Geometry: see drawing. Coordinates: mm, zero at the bounding-box minimum. A direction names the side the tool comes from. Give positions to 0.01 mm unless a question says otherwise; leave off trailing zeros. Write each loop counter-clockwise with the first axis right and the second up, starting at its lowest first coordinate (ties: lowest second). Pieces come first, ordered by that corner, then holes. Notation, with made-up numbers: (-39, 76) -> (-5, 76) arc R36 ccw to (-5, 112) -> close; hole circle Ø2 at (35.5, 31.25). An arc over 180 degrees is marked (long way). Answer as a JSON object with one key per item and string values. Group by question number.
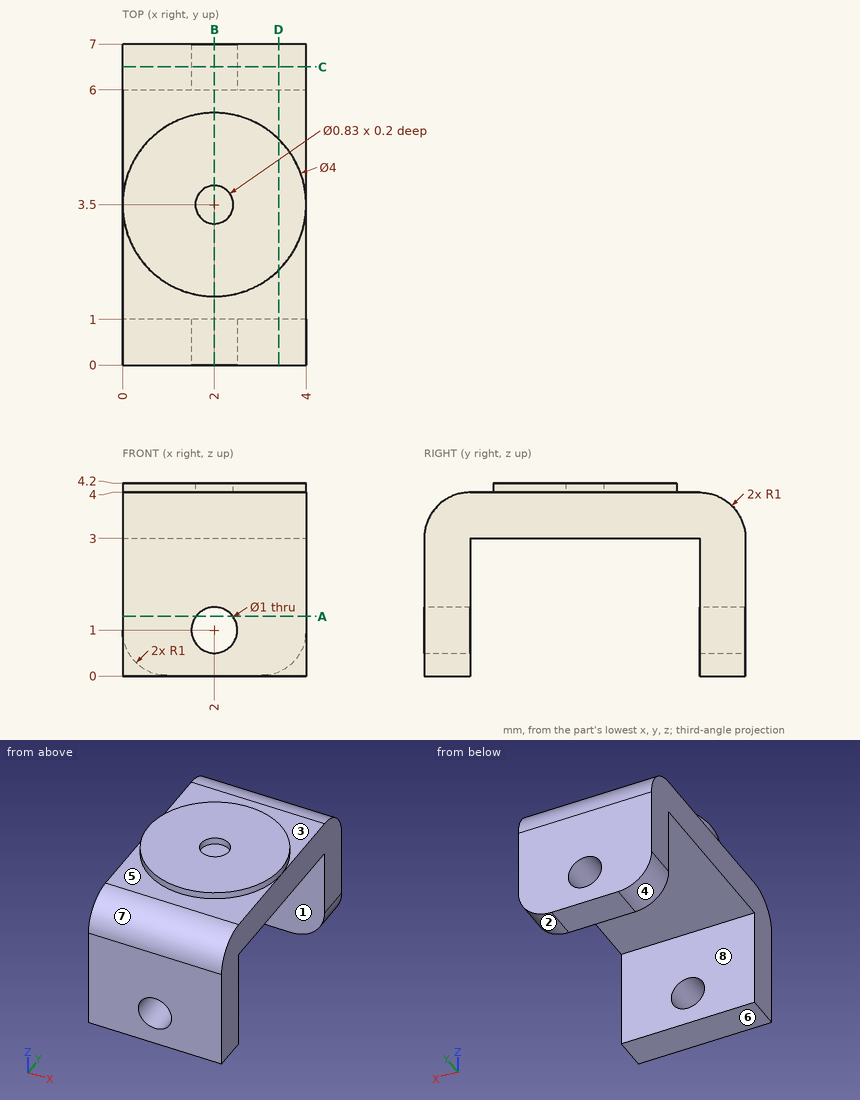
1. Line query: line 1 (Y direction, x = 0.65, z = 2.4); line 2 (Y direction, x = 2, z = 4.15) (3 decimals); line 3 (X direction, y = 0.65, z = 1). Output: solid intervals per line, ascending.
2. Contact query for flat-ended pins moving along their axis: pin 1 Ø1.2 at (x, y) = (1, 4) entering from -Z; pin 2 Ø2 at (y, z) = (4, 1.5) entering from +X. Output: stop coordinate, or through.
3. Mould query, pull axis Y, two halves, no side actions, for the marked faces 6, 7 and 8. Classes: pulls with the +Y half, pulls with the -Y half, needs draft (parallel to the pull), parting line crosses it, or undercut.
4. Reachability of the marked faces 1, 2, 3, 4 and 5 from +Z, -Z, +X, -X, +Y, -Y: full face, straight path, thin tool, end or side. Return the list, or none.
5. Section A-A (z = 1.3). Return the cut outline in (x, y).
6. Section D-D (x = 3.4). Return the cut outline in (y, z), plus the area to 3 significant figures.
7. Section C-C (y = 6.5). Return the cut outline in (x, z), plus the area to 3 significant figures.
8. Section B-B (x = 2). Return the cut outline in (y, z) (3 decimals), plus the area to 3 significant figures.
Working result:
{
 "1": {"line 1": "y = 0 to 1, 6 to 7", "line 2": "y = 1.5 to 3.085, 3.915 to 5.5", "line 3": "x = 0 to 1.5, 2.5 to 4"},
 "2": {"pin 1": "stops at z = 3", "pin 2": "passes through"},
 "3": {"face 6": "needs draft", "face 7": "pulls with the -Y half", "face 8": "undercut"},
 "4": {"face 1": "-Z, +X, -X", "face 2": "-Z, +X, +Y", "face 3": "+Z, +Y", "face 4": "-Z, -X, +Y", "face 5": "+Z, -Y"},
 "5": {"outline": "(0, 0) -> (1.6, 0) -> (1.6, 1) -> (0, 1) -> close; (0, 6) -> (1.6, 6) -> (1.6, 7) -> (0, 7) -> close; (2.4, 0) -> (4, 0) -> (4, 1) -> (2.4, 1) -> close; (2.4, 6) -> (4, 6) -> (4, 7) -> (2.4, 7) -> close"},
 "6": {"outline": "(0, 0) -> (1, 0) -> (1, 3) -> (6, 3) -> (6, 0.08) -> (7, 0.08) -> (7, 3) arc R1 ccw to (6, 4) -> (4.93, 4) -> (4.93, 4.2) -> (2.07, 4.2) -> (2.07, 4) -> (1, 4) arc R1 ccw to (0, 3) -> close", "area": "13.1 mm^2"},
 "7": {"outline": "(0, 1) arc R1 ccw to (1, 0) -> (3, 0) arc R1 ccw to (4, 1) -> (4, 3.87) -> (0, 3.87) -> close; hole circle Ø1 at (2, 1)", "area": "14.2 mm^2"},
 "8": {"outline": "(0, 0) -> (1, 0) -> (1, 0.5) -> (0, 0.5) -> close; (0, 1.5) -> (1, 1.5) -> (1, 3) -> (6, 3) -> (6, 1.5) -> (7, 1.5) -> (7, 3) arc R1 ccw to (6, 4) -> (5.5, 4) -> (5.5, 4.2) -> (3.915, 4.2) -> (3.915, 4) -> (3.085, 4) -> (3.085, 4.2) -> (1.5, 4.2) -> (1.5, 4) -> (1, 4) arc R1 ccw to (0, 3) -> close; (6, 0) -> (7, 0) -> (7, 0.5) -> (6, 0.5) -> close", "area": "11.2 mm^2"}
}
